For this review, take the finished solid that the model builds, in its own axes (mm). A direction names the side the tool comes from. Give positions to 0.01 mm unless a question says otherwise; leave off trailing zeros. Loops run counter-clockwise (first coordinate to the right, second up) from the corner with the lowest first, then second, coordinate; pieces in that order, holes last.
```python
from build123d import *

# Parameters (mm, degrees)
SKETCH1_W                = 25
SKETCH1_H                = 45
BOSS_EXTRUDE1_DEPTH      = 30
CUT_EXTRUDE1_REACH       = 61.582
SKETCH2_R                = 6
CUT_EXTRUDE10_DEPTH      = 5
CUT_EXTRUDE11_DEPTH      = 60.581876439
CUT_EXTRUDE11_DEPTH_BACK = 60.581876439
CUT_EXTRUDE23_START      = -20
SKETCH9_R                = 3
CUT_EXTRUDE23_DEPTH      = 2
FILLET1_R                = 1


with BuildPart() as part:
    # Sketch1 → Boss-Extrude1 (new body)
    with BuildSketch(Plane.XY):
        with Locations((12.5, 22.5)):
            Rectangle(SKETCH1_W, SKETCH1_H)
    extrude(amount=BOSS_EXTRUDE1_DEPTH)

    # Sketch2 → Cut-Extrude1 (cut, up to next)
    with BuildSketch(Plane.XY.offset(30), mode=Mode.PRIVATE) as cut_extrude1_sk1:
        with Locations((12.5, 12.5)):
            Circle(SKETCH2_R)
    cut_extrude1_tool1 = extrude(cut_extrude1_sk1.sketch, amount=-CUT_EXTRUDE1_REACH, mode=Mode.PRIVATE) & part.part
    # Sketch2 → Cut-Extrude1 (cut, up to next)
    with BuildSketch(Plane.XY.offset(30), mode=Mode.PRIVATE) as cut_extrude1_sk2:
        with Locations((12.5, 32.5)):
            Circle(SKETCH2_R)
    cut_extrude1_tool2 = extrude(cut_extrude1_sk2.sketch, amount=-CUT_EXTRUDE1_REACH, mode=Mode.PRIVATE) & part.part
    add(cut_extrude1_tool1.solids().sort_by_distance((12.5, 12.5, 30))[0], mode=Mode.SUBTRACT)
    add(cut_extrude1_tool2.solids().sort_by_distance((12.5, 32.5, 30))[0], mode=Mode.SUBTRACT)

    # Sketch3 → Cut-Extrude10 (cut)
    with BuildSketch(Plane(origin=(25, 0, 0), x_dir=(0, 0, -1), z_dir=(1, 0, 0))):
        with BuildLine():
            Line((-12, 32.5), (-12, 26.5))
            ThreePointArc((-12, 26.5), (-10, 22.5), (-12, 18.5))
            Line((-12, 18.5), (-12, 12.5))
            ThreePointArc((-12, 12.5), (-15, 9.5), (-18, 12.5))
            Line((-18, 12.5), (-18, 18.5))
            ThreePointArc((-18, 18.5), (-20, 22.5), (-18, 26.5))
            Line((-18, 26.5), (-18, 32.5))
            ThreePointArc((-18, 32.5), (-15, 35.5), (-12, 32.5))
        make_face()
    extrude(amount=-CUT_EXTRUDE10_DEPTH, mode=Mode.SUBTRACT)

    # Sketch8 → Cut-Extrude11 (cut, two sides: drawn at the far end of the back side and taken through both)
    with BuildSketch(Plane.XY.offset(30).offset(-CUT_EXTRUDE11_DEPTH_BACK)):
        Polygon((7, 45), (0, 40), (0, 45), align=None)
        Polygon((0, 0), (7, 0), (0, 5), align=None)
        Polygon((25, 45), (25, 40), (18, 45), align=None)
        Polygon((25, 5), (18, 0), (25, 0), align=None)
    extrude(amount=CUT_EXTRUDE11_DEPTH + CUT_EXTRUDE11_DEPTH_BACK, mode=Mode.SUBTRACT)

    # Sketch9 → Cut-Extrude23 (cut)
    with BuildSketch(Plane.ZY.offset(CUT_EXTRUDE23_START)):
        with Locations(Location((15, 22.5, 0), (0, 0, 180))):
            Circle(SKETCH9_R)
    extrude(amount=CUT_EXTRUDE23_DEPTH, mode=Mode.SUBTRACT)

    # Fillet1
    fillet1_edges = [part.edges().sort_by_distance(p)[0] for p in [
        (6.5, 12.5, 0),
        (6.5, 12.5, 30),
        (6.5, 32.5, 0),
        (6.5, 32.5, 30),
        (0, 22.5, 0),
        (12.5, 45, 0),
        (25, 22.5, 0),
        (12.5, 0, 0),
        (0, 22.5, 30),
        (12.5, 0, 30),
        (25, 22.5, 30),
        (12.5, 45, 30),
        (18, 45, 15),
        (25, 40, 15),
        (21.5, 42.5, 30),
        (21.5, 42.5, 0),
        (0, 5, 15),
        (3.5, 2.5, 30),
        (3.5, 2.5, 0),
        (7, 0, 15),
        (18, 0, 15),
        (21.5, 2.5, 30),
        (21.5, 2.5, 0),
        (25, 5, 15),
        (0, 40, 15),
        (7, 45, 15),
        (3.5, 42.5, 30),
        (3.5, 42.5, 0),
    ]]
    fillet(fillet1_edges, radius=FILLET1_R)


solid = part.part
```
Q1. Consider section A-A on x = 12.5. Give the boundary of the cut face in (y, z).
Answers:
outline: (0, 1) arc R1 ccw to (1, 0) - (5.5, 0) arc R1 ccw to (6.5, 1) - (6.5, 29) arc R1 ccw to (5.5, 30) - (1, 30) arc R1 ccw to (0, 29) - close; (18.5, 1) arc R1 ccw to (19.5, 0) - (25.5, 0) arc R1 ccw to (26.5, 1) - (26.5, 29) arc R1 ccw to (25.5, 30) - (19.5, 30) arc R1 ccw to (18.5, 29) - close; (38.5, 1) arc R1 ccw to (39.5, 0) - (44, 0) arc R1 ccw to (45, 1) - (45, 29) arc R1 ccw to (44, 30) - (39.5, 30) arc R1 ccw to (38.5, 29) - close
Q2. Consider section D-D on z = 15. Give the boundary of the cut face in (x, y).
Answers:
outline: (0, 5.51) arc R1 ccw to (0.42, 4.7) - (6.74, 0.19) arc R1 ccw to (7.32, 0) - (17.68, 0) arc R1 ccw to (18.26, 0.19) - (24.58, 4.7) arc R1 ccw to (25, 5.51) - (25, 9.5) - (20, 9.5) - (20, 19.5) - (18, 19.5) - (18, 25.5) - (20, 25.5) - (20, 35.5) - (25, 35.5) - (25, 39.49) arc R1 ccw to (24.58, 40.3) - (18.26, 44.81) arc R1 ccw to (17.68, 45) - (7.32, 45) arc R1 ccw to (6.74, 44.81) - (0.42, 40.3) arc R1 ccw to (0, 39.49) - close; hole circle Ø12 at (12.5, 12.5); hole circle Ø12 at (12.5, 32.5)
Q3. Consider section C-C on y = 22.5. Give the boundary of the cut face in (x, z), plus the area to 3 significant figures.
Answers:
outline: (0, 1) arc R1 ccw to (1, 0) - (24, 0) arc R1 ccw to (25, 1) - (25, 10) - (20, 10) - (20, 12) - (18, 12) - (18, 18) - (20, 18) - (20, 20) - (25, 20) - (25, 29) arc R1 ccw to (24, 30) - (1, 30) arc R1 ccw to (0, 29) - close
area: 687 mm2
Q4. For pin 1 Ø3 at (y, z) = (23, 13.5) entering from +X; pin 2 Ø1 at (x, z) = (3, 13.5) entering from -Y; pin 3 Ø11 at (x, y) = (12.5, 32.5) entering from -Z; pin 4 Ø3 at (x, z) = (21, 17) entering from -Y, all flat-tipped, find the tip position at first contact; note any pin that passes through.
Answers:
pin 1: stops at x = 20
pin 2: stops at y = 2.5
pin 3: passes through
pin 4: stops at y = 1.07
Q5. Machinability: for faces 4 (the flat face through (21.5, 2.5, 14.8)), 5 (the cylindrical face through (19, 24.3, 17.4)), which of the approach directions +Z, -Z, +X, -X, +Y, -Y give a long, thin tool a straight path to every point of the face, cutting with its end or side? Answer none if there is none.
Answers:
face 4: +Z, -Z, +X, -Y
face 5: +X
Q6. Consider section B-B on z = 11. Give the boundary of the cut face in (x, y).
Answers:
outline: (0, 5.51) arc R1 ccw to (0.42, 4.7) - (6.74, 0.19) arc R1 ccw to (7.32, 0) - (17.68, 0) arc R1 ccw to (18.26, 0.19) - (24.58, 4.7) arc R1 ccw to (25, 5.51) - (25, 19.5) - (20, 19.5) - (20, 25.5) - (25, 25.5) - (25, 39.49) arc R1 ccw to (24.58, 40.3) - (18.26, 44.81) arc R1 ccw to (17.68, 45) - (7.32, 45) arc R1 ccw to (6.74, 44.81) - (0.42, 40.3) arc R1 ccw to (0, 39.49) - close; hole circle Ø12 at (12.5, 12.5); hole circle Ø12 at (12.5, 32.5)
Q7. For probe 1 along Y at (x, z) = (12.5, 7.25); probe 2 along Y at (x, z) = (11.5, 8.25); probe 3 along Z at (x, y) = (19.45, 22.5), list the stretches that pass through material, from the lowest coordinate up.
Answers:
probe 1: y = 0 to 6.5, 18.5 to 26.5, 38.5 to 45
probe 2: y = 0 to 6.58, 18.42 to 26.58, 38.42 to 45
probe 3: z = 0 to 12, 18 to 30
Q8. Mouldability with a two-part tool opening along Y and no side actions: class faces 1 (the flat face through (21.5, 42.5, 14.8)), 2 (the flat face through (18, 22, 15)), 3 (the flat face through (0, 22, 15)) as +Y half, -Y half, draft (parallel to the pull), parting line (faces both ways), or undercut.
Answers:
face 1: +Y half
face 2: undercut
face 3: draft
